Verification items for the finished model (mm, model axes). A direction names the side the tool comes from. Coordinates: 2 decimals unless noted, no trailing zeros. Loops run counter-clockwise (first coordinate to the right, second up) from the corner with the lowest first, then second, coordinate; pieces in that order, holes last.
Q1. Access from +Z, -Z, +X, -X, +Y, -Y to the whole of each face (thin tool, end or side, straight path). Record for faces 1 (the face through (53, 5, -1)), 2 (the face through (-40, 3, -30)), 3 (the face through (2.025, 5, 29)).
Q2. Material ranges on probe 1 along Z at (x, y) = (-30.5, 4.75) (3 decimals); probe 2 along X at (y, z) = (5, -7) (1 decimal); probe 3 along X at (y, z) = (5.75, 25) (1 decimal), recorded low to high.
Q3. Mould release check, pull along Z, two halves, no side actions. Record for faces 4 (the face through (-49.692, 5.226, 49.863)), 5 (the face through (-21.078, 5, -10)), 6 (the face through (0, 9.8, -51)): +Z half, -Z half, draft (parallel to the pull), parting line (faces both ways), or undercut.
Q4. Sectioned sample at A-A (z = -4). Enter the section's corners in (x, y) (1 decimal), then the cut area to 3 significant figures.
Q5. Go/stop test with flat-tipped pins: P1, Ø4.5, axis at x = 10.5, z = -25, coming from the +Y side; P2, Ø1, axis at x = 2, z = -17.5, coming from the +Y side. Record where each tip stops, or that it passes through.
Q6. Sectioned sample at B-B (x = 0.5). Enter the section's corners in (y, z).
Q7. Sectioned sample at C-C (y = 1.5). Count the separate pieces of the cut face and the enclosed holes in it, then the cut area to 3 significant figures.
Autodesk Fusion 360 part; units mm, degrees
sketch "Sketch1" plane through (0, 0, 0) normal (0, 1, 0) x (1, 0, 0)
  line L0 (0, 0) -> (0, 32) construction
  line L1 (0, 0) -> (-33, 0) construction
  line L2 (-42, 53) -> (42, 53)
  line L3 (53, 42) -> (53, -42)
  line L4 (42, -53) -> (-42, -53)
  line L5 (-53, -42) -> (-53, 42)
  arc A0 (-42, 53) -> (-53, 42) centre (-42, 42) ccw
  arc A1 (-53, -42) -> (-42, -53) centre (-42, -42) ccw
  arc A2 (42, -53) -> (53, -42) centre (42, -42) ccw
  arc A3 (53, 42) -> (42, 53) centre (42, 42) ccw
  point P0 (-53, 53)
  point P1 (53, 53)
  dimension "d1" = 106
  dimension "d2" = 11
  dimension "d49" = 106
extrude "Extrude1" add sketch "Sketch1" along normal blind 10.6
sketch "Sketch2" plane through (0, 10.6, 0) normal (0, 1, 0) x (-1, 0, 0)
  arc A0 (-42, 53) -> (-53, 42) centre (-42, 42) ccw
  line L0 (-53, 42) -> (-53, -42)
  arc A1 (-53, -42) -> (-42, -53) centre (-42, -42) ccw
  line L1 (-42, -53) -> (42, -53)
  arc A2 (42, -53) -> (53, -42) centre (42, -42) ccw
  line L2 (53, -42) -> (53, 42)
  arc A3 (53, 42) -> (42, 53) centre (42, 42) ccw
  line L3 (42, 53) -> (-42, 53)
  line L4 (48, -42) -> (48, 42)
  arc A4 (48, 42) -> (42, 48) centre (42, 42) ccw
  line L5 (42, 48) -> (-42, 48)
  arc A5 (-42, 48) -> (-48, 42) centre (-42, 42) ccw
  line L6 (-48, 42) -> (-48, -42)
  arc A6 (-48, -42) -> (-42, -48) centre (-42, -42) ccw
  line L7 (-42, -48) -> (42, -48)
  arc A7 (42, -48) -> (48, -42) centre (42, -42) ccw
  dimension "d5" = -5
extrude "Extrude2" cut sketch "Sketch2" against normal blind 2 contours L4 A4 L5 A5 L6 A6 L7 A7
sketch "Sketch3" plane through (0, 8.6, 0) normal (0, 1, 0) x (-1, 0, 0)
  arc A0 (42, -48) -> (48, -42) centre (42, -42) ccw
  line L0 (48, -42) -> (48, 42)
  arc A1 (48, 42) -> (42, 48) centre (42, 42) ccw
  line L1 (42, 48) -> (-42, 48)
  arc A2 (-42, 48) -> (-48, 42) centre (-42, 42) ccw
  line L2 (-48, 42) -> (-48, -42)
  arc A3 (-48, -42) -> (-42, -48) centre (-42, -42) ccw
  line L3 (-42, -48) -> (42, -48)
  line L4 (46, -42) -> (46, 42)
  arc A4 (46, 42) -> (42, 46) centre (42, 42) ccw
  line L5 (42, 46) -> (-42, 46)
  arc A5 (-42, 46) -> (-46, 42) centre (-42, 42) ccw
  line L6 (-46, 42) -> (-46, -42)
  arc A6 (-46, -42) -> (-42, -46) centre (-42, -42) ccw
  line L7 (-42, -46) -> (42, -46)
  arc A7 (42, -46) -> (46, -42) centre (42, -42) ccw
  dimension "d8" = -2
extrude "Extrude3" cut sketch "Sketch3" against normal blind 2.2 contours L4 A4 L5 A5 L6 A6 L7 A7
sketch "Sketch5" plane through (0, 6.4, 0) normal (0, 1, 0) x (-1, 0, 0)
  arc A0 (42, -46) -> (46, -42) centre (42, -42) ccw
  line L0 (46, -42) -> (46, 42)
  arc A1 (46, 42) -> (42, 46) centre (42, 42) ccw
  line L1 (42, 46) -> (-42, 46)
  arc A2 (-42, 46) -> (-46, 42) centre (-42, 42) ccw
  line L2 (-46, 42) -> (-46, -42)
  arc A3 (-46, -42) -> (-42, -46) centre (-42, -42) ccw
  line L3 (-42, -46) -> (42, -46)
  line L4 (0, 0) -> (0, -26) construction
  line L5 (0, 0) -> (25, 0) construction
  line L6 (-2.025, -36.075) -> (-17.025, -36.075)
  line L7 (-17.025, -36.075) -> (-17.025, -21.075)
  line L8 (-17.025, -21.075) -> (-2.025, -21.075)
  line L9 (-2.025, -21.075) -> (-2.025, -36.075)
  line L10 (17.025, -36.075) -> (2.025, -36.075)
  line L11 (2.025, -36.075) -> (2.025, -21.075)
  line L12 (2.025, -21.075) -> (17.025, -21.075)
  line L13 (17.025, -21.075) -> (17.025, -36.075)
  line L14 (-21.075, -17.025) -> (-36.075, -17.025)
  line L15 (-36.075, -17.025) -> (-36.075, -2.025)
  line L16 (-36.075, -2.025) -> (-21.075, -2.025)
  line L17 (-21.075, -2.025) -> (-21.075, -17.025)
  line L18 (-2.025, -17.025) -> (-17.025, -17.025)
  line L19 (-17.025, -17.025) -> (-17.025, -2.025)
  line L20 (-17.025, -2.025) -> (-2.025, -2.025)
  line L21 (-2.025, -2.025) -> (-2.025, -17.025)
  line L22 (17.025, -17.025) -> (2.025, -17.025)
  line L23 (2.025, -17.025) -> (2.025, -2.025)
  line L24 (2.025, -2.025) -> (17.025, -2.025)
  line L25 (17.025, -2.025) -> (17.025, -17.025)
  line L26 (36.0775, -17.025) -> (21.0775, -17.025)
  line L27 (21.0775, -17.025) -> (21.0775, -2.025)
  line L28 (21.0775, -2.025) -> (36.0775, -2.025)
  line L29 (36.0775, -2.025) -> (36.0775, -17.025)
  line L30 (-21.075, 2.025) -> (-36.075, 2.025)
  line L31 (-36.075, 2.025) -> (-36.075, 17.025)
  line L32 (-36.075, 17.025) -> (-21.075, 17.025)
  line L33 (-21.075, 17.025) -> (-21.075, 2.025)
  line L34 (-2.025, 2.025) -> (-17.025, 2.025)
  line L35 (-17.025, 2.025) -> (-17.025, 17.025)
  line L36 (-17.025, 17.025) -> (-2.025, 17.025)
  line L37 (-2.025, 17.025) -> (-2.025, 2.025)
  line L38 (17.025, 2.025) -> (2.025, 2.025)
  line L39 (2.025, 2.025) -> (2.025, 17.025)
  line L40 (2.025, 17.025) -> (17.025, 17.025)
  line L41 (17.025, 17.025) -> (17.025, 2.025)
  line L42 (36.0775, 2.025) -> (21.0775, 2.025)
  line L43 (21.0775, 2.025) -> (21.0775, 17.025)
  line L44 (21.0775, 17.025) -> (36.0775, 17.025)
  line L45 (36.0775, 17.025) -> (36.0775, 2.025)
  line L46 (36.0775, 21.075) -> (21.0775, 21.075)
  line L47 (21.0775, 21.075) -> (21.0775, 36.075)
  line L48 (21.0775, 36.075) -> (36.0775, 36.075)
  line L49 (36.0775, 36.075) -> (36.0775, 21.075)
  line L50 (-2.025, 21.075) -> (-17.025, 21.075)
  line L51 (-17.025, 21.075) -> (-17.025, 36.075)
  line L52 (-17.025, 36.075) -> (-2.025, 36.075)
  line L53 (-2.025, 36.075) -> (-2.025, 21.075)
  line L54 (17.025, 21.075) -> (2.025, 21.075)
  line L55 (2.025, 21.075) -> (2.025, 36.075)
  line L56 (2.025, 36.075) -> (17.025, 36.075)
  line L57 (17.025, 36.075) -> (17.025, 21.075)
  line L58 (9.525, -36.075) -> (9.525, -21.075) construction
  line L59 (17.025, -28.575) -> (2.025, -28.575) construction
  line L60 (28.5775, -17.025) -> (28.5775, -2.025) construction
  line L61 (36.0775, -9.525) -> (21.0775, -9.525) construction
  line L62 (-2.025, 9.525) -> (-17.025, 9.525) construction
  line L63 (-9.525, 2.025) -> (-9.525, 17.025) construction
  line L64 (36.0775, 28.575) -> (21.0775, 28.575) construction
  dimension "d16" = 9.525
  dimension "d17" = 28.575
  dimension "d18" = 9.525
  dimension "d19" = 28.575
  dimension "d20" = 28.5775
  dimension "d21" = 9.525
  dimension "d23" = 15
  dimension "d24" = 9.525
extrude "Extrude5" cut sketch "Sketch5" against normal blind 3.1 contours L6 L7 L8 L9 | L10 L11 L12 L13 | L14 L15 L16 L17 | L18 L19 L20 L21 | L22 L23 L24 L25 | L26 L27 L28 L29 | L30 L31 L32 L33 | L34 L35 L36 L37 | L38 L39 L40 L41 | L42 L43 L44 L45 | L46 L47 L48 L49 | L50 L51 L52 L53 | L54 L55 L56 L57
sketch "Sketch6" plane through (0, 3.3, 0) normal (0, 1, 0) x (-1, 0, 0)
  line L0 (17.025, -21.075) -> (2.025, -21.075)
  line L1 (2.025, -21.075) -> (2.025, -36.075)
  line L2 (2.025, -36.075) -> (17.025, -36.075)
  line L3 (17.025, -36.075) -> (17.025, -21.075)
  line L4 (9.525, -36.075) -> (9.525, -21.075) construction
  line L5 (17.025, -28.575) -> (2.025, -28.575) construction
  circle A0 centre (9.525, -28.575) radius 3.5
  circle A1 centre (-9.525, -28.575) radius 3.5
  circle A2 centre (28.575, -9.525) radius 3.5
  circle A3 centre (9.525, -9.525) radius 3.5
  circle A4 centre (-9.525, -9.525) radius 3.5
  circle A5 centre (-28.575, -9.525) radius 3.5
  circle A6 centre (-28.575, 9.525) radius 3.5
  circle A7 centre (-9.525, 9.525) radius 3.5
  circle A8 centre (9.525, 9.525) radius 3.5
  circle A9 centre (28.575, 9.525) radius 3.5
  circle A10 centre (9.525, 28.575) radius 3.5
  circle A11 centre (-9.525, 28.575) radius 3.5
  circle A12 centre (28.575, 28.575) radius 3.5
  line L6 (46, -9.525) -> (-46, -9.525) construction
  line L7 (46, 9.525) -> (-46, 9.525) construction
  line L8 (28.575, -46) -> (28.575, 46) construction
  line L9 (-9.525, -46) -> (-9.525, 46) construction
  line L10 (-28.575, -46) -> (-28.575, 46) construction
  line L11 (46, 28.575) -> (-46, 28.575) construction
  line L12 (42, -46) -> (-42, -46)
  line L13 (-42, 46) -> (42, 46)
  line L14 (-46, -42) -> (-46, 42)
  line L15 (46, 42) -> (46, -42)
  dimension "d27" = 7
  dimension "d28" = 28.575
  dimension "d29" = 9.525
  dimension "d30" = 9.525
  dimension "d31" = 9.525
  dimension "d32" = 28.575
  dimension "d33" = 28.575
extrude "Extrude6" cut sketch "Sketch6" against normal up to surface (3.3 mm away) contours A0 | A1 | A2 | A3 | A4 | A5 | A6 | A7 | A8 | A9 | A10 | A11 | A12
sketch "Sketch7" plane through (0, 6.4, 0) normal (0, 1, 0) x (-1, 0, 0)
  arc A0 (42, -46) -> (46, -42) centre (42, -42) ccw
  line L0 (46, -42) -> (46, 42)
  arc A1 (46, 42) -> (42, 46) centre (42, 42) ccw
  line L1 (42, 46) -> (-42, 46)
  arc A2 (-42, 46) -> (-46, 42) centre (-42, 42) ccw
  line L2 (-46, 42) -> (-46, -42)
  arc A3 (-46, -42) -> (-42, -46) centre (-42, -42) ccw
  line L3 (-42, -46) -> (42, -46)
  line L4 (21.0775, 21.075) -> (21.0775, 36.075)
  line L5 (21.0775, 36.075) -> (36.0775, 36.075)
  line L6 (36.0775, 36.075) -> (36.0775, 21.075)
  line L7 (36.0775, 21.075) -> (21.0775, 21.075)
  line L8 (2.025, 2.025) -> (2.025, 17.025)
  line L9 (2.025, 17.025) -> (17.025, 17.025)
  line L10 (17.025, 17.025) -> (17.025, 2.025)
  line L11 (17.025, 2.025) -> (2.025, 2.025)
  line L12 (-17.025, -17.025) -> (-17.025, -2.025)
  line L13 (-17.025, -2.025) -> (-2.025, -2.025)
  line L14 (-2.025, -2.025) -> (-2.025, -17.025)
  line L15 (-2.025, -17.025) -> (-17.025, -17.025)
  line L16 (2.025, -36.075) -> (2.025, -21.075)
  line L17 (2.025, -21.075) -> (17.025, -21.075)
  line L18 (17.025, -21.075) -> (17.025, -36.075)
  line L19 (17.025, -36.075) -> (2.025, -36.075)
  line L20 (2.025, -17.025) -> (2.025, -2.025)
  line L21 (2.025, -2.025) -> (17.025, -2.025)
  line L22 (17.025, -2.025) -> (17.025, -17.025)
  line L23 (17.025, -17.025) -> (2.025, -17.025)
  line L24 (-17.025, 2.025) -> (-17.025, 17.025)
  line L25 (-17.025, 17.025) -> (-2.025, 17.025)
  line L26 (-2.025, 17.025) -> (-2.025, 2.025)
  line L27 (-2.025, 2.025) -> (-17.025, 2.025)
  line L28 (-17.025, 21.075) -> (-17.025, 36.075)
  line L29 (-17.025, 36.075) -> (-2.025, 36.075)
  line L30 (-2.025, 36.075) -> (-2.025, 21.075)
  line L31 (-2.025, 21.075) -> (-17.025, 21.075)
  line L32 (21.0775, 2.025) -> (21.0775, 17.025)
  line L33 (21.0775, 17.025) -> (36.0775, 17.025)
  line L34 (36.0775, 17.025) -> (36.0775, 2.025)
  line L35 (36.0775, 2.025) -> (21.0775, 2.025)
  line L36 (-36.075, -17.025) -> (-36.075, -2.025)
  line L37 (-36.075, -2.025) -> (-21.075, -2.025)
  line L38 (-21.075, -2.025) -> (-21.075, -17.025)
  line L39 (-21.075, -17.025) -> (-36.075, -17.025)
  line L40 (-17.025, -36.075) -> (-17.025, -21.075)
  line L41 (-17.025, -21.075) -> (-2.025, -21.075)
  line L42 (-2.025, -21.075) -> (-2.025, -36.075)
  line L43 (-2.025, -36.075) -> (-17.025, -36.075)
  line L44 (21.0775, -17.025) -> (21.0775, -2.025)
  line L45 (21.0775, -2.025) -> (36.0775, -2.025)
  line L46 (36.0775, -2.025) -> (36.0775, -17.025)
  line L47 (36.0775, -17.025) -> (21.0775, -17.025)
  line L48 (-36.075, 2.025) -> (-36.075, 17.025)
  line L49 (-36.075, 17.025) -> (-21.075, 17.025)
  line L50 (-21.075, 17.025) -> (-21.075, 2.025)
  line L51 (-21.075, 2.025) -> (-36.075, 2.025)
  line L52 (2.025, 21.075) -> (2.025, 36.075)
  line L53 (2.025, 36.075) -> (17.025, 36.075)
  line L54 (17.025, 36.075) -> (17.025, 21.075)
  line L55 (17.025, 21.075) -> (2.025, 21.075)
  line L56 (-20.575, -36.575) -> (-36.575, -36.575)
  line L57 (-36.575, -36.575) -> (-36.575, -20.575)
  line L58 (-36.575, -20.575) -> (-20.575, -20.575)
  line L59 (-20.575, -20.575) -> (-20.575, -36.575)
  line L60 (40, -42) -> (17.625, -42)
  line L61 (17.625, -42) -> (17.625, -19.025)
  line L62 (17.625, -19.025) -> (40, -19.025)
  line L63 (40, -19.025) -> (40, -42)
  line L64 (-28.575, -36.575) -> (-28.575, -20.575) construction
  line L65 (-20.575, -28.575) -> (-36.575, -28.575) construction
  dimension "d36" = 16
  dimension "d37" = 4
  dimension "d40" = 28.575
  dimension "d43" = 6
  dimension "d44" = 28.575
  dimension "d50" = 0.6
  dimension "d54" = 2
extrude "Extrude7" cut sketch "Sketch7" against normal up to surface (6.4 mm away) contours L56 L57 L58 L59 | L60 L61 L62 L63
sketch "Sketch8" plane through (0, 0, -53) normal (0, 0, -1) x (-1, 0, 0)
  line L0 (-42, 0) -> (42, 0)
  line L1 (42, 0) -> (42, 10.6)
  line L2 (42, 10.6) -> (-42, 10.6)
  line L3 (-42, 10.6) -> (-42, 0)
  line L4 (0, 0) -> (0, 10.6) construction
  line L5 (6, 10.6) -> (-6, 10.6)
  line L6 (-6, 10.6) -> (-6, 9.8)
  line L7 (-6, 9.8) -> (6, 9.8)
  line L8 (6, 9.8) -> (6, 10.6)
  dimension "d45" = 0.8
  dimension "d46" = 12
extrude "Extrude8" cut sketch "Sketch8" against normal up to surface (5 mm away) contours L2 L5 L6 L7 L8
Geometry check:
1. face 1: +Z, -Z, +X, +Y, -Y
1. face 2: +Y, -Y
1. face 3: +Y
2. probe 1: z = -53 to -42, -19.025 to -17.025, -2.025 to 2.025, 17.025 to 21.075, 36.075 to 53
2. probe 2: x = -53 to -36.1, -21.1 to -17, -2 to 2, 17 to 21.1, 36.1 to 53
2. probe 3: x = -53 to -36.1, -21.1 to -17, -2 to 2, 17 to 53
3. face 4: +Z half
3. face 5: undercut
3. face 6: draft
4. outline: (-53, 0) - (53, 0) - (53, 10.6) - (48, 10.6) - (48, 8.6) - (46, 8.6) - (46, 6.4) - (36.1, 6.4) - (36.1, 3.3) - (21.1, 3.3) - (21.1, 6.4) - (17, 6.4) - (17, 3.3) - (2, 3.3) - (2, 6.4) - (-2, 6.4) - (-2, 3.3) - (-17, 3.3) - (-17, 6.4) - (-21.1, 6.4) - (-21.1, 3.3) - (-36.1, 3.3) - (-36.1, 6.4) - (-46, 6.4) - (-46, 8.6) - (-48, 8.6) - (-48, 10.6) - (-53, 10.6) - close
4. area: 543 mm2
5. P1: stops at y = 3.3
5. P2: stops at y = 6.4
6. outline: (0, -53) - (9.8, -53) - (9.8, -48) - (8.6, -48) - (8.6, -46) - (6.4, -46) - (6.4, 46) - (8.6, 46) - (8.6, 48) - (10.6, 48) - (10.6, 53) - (0, 53) - close
7. separate pieces: 1
7. enclosed holes: 15
7. area: 9,860 mm2
